```python
from build123d import *

# Parameters (mm, degrees)
SKETCH1_R               = 3
BOSS_EXTRUDE1_DEPTH     = 98.5
SKETCH2_R               = 4
BOSS_EXTRUDE2_DEPTH     = 4.7
SKETCH3_R               = 9
BOSS_EXTRUDE3_DEPTH     = 7.9
SKETCH4_R               = 5.9
BOSS_EXTRUDE4_DEPTH     = 8
SKETCH5_R               = 9
BOSS_EXTRUDE5_DEPTH     = 3
SKETCH6_R               = 1.4
CUT_EXTRUDE1_DEPTH      = 82
CUT_EXTRUDE1_DEPTH_BACK = 82
SKETCH7_R               = 3
SKETCH7_R_2             = 0.75
CUT_EXTRUDE2_DEPTH      = 9


with BuildPart() as part:
    # Sketch1 → Boss-Extrude1 (new body)
    with BuildSketch(Plane.XY):
        Circle(SKETCH1_R)
    extrude(amount=BOSS_EXTRUDE1_DEPTH)

    # Sketch2 → Boss-Extrude2 (add)
    with BuildSketch(Plane.XY.offset(98.5)):
        Circle(SKETCH2_R)
    extrude(amount=BOSS_EXTRUDE2_DEPTH)

    # Sketch3 → Boss-Extrude3 (add)
    with BuildSketch(Plane.XY.offset(103.2)):
        Circle(SKETCH3_R)
    extrude(amount=BOSS_EXTRUDE3_DEPTH)

    # Sketch4 → Boss-Extrude4 (add)
    with BuildSketch(Plane.XY.offset(111.1)):
        Circle(SKETCH4_R)
    extrude(amount=BOSS_EXTRUDE4_DEPTH)

    # Sketch5 → Boss-Extrude5 (add)
    with BuildSketch(Plane.XY.offset(119.1)):
        Circle(SKETCH5_R)
    extrude(amount=BOSS_EXTRUDE5_DEPTH)

    # Sketch6 → Cut-Extrude1 (cut, two sides)
    with BuildSketch(Plane(origin=(0, 0, 0), x_dir=(1, 0, 0), z_dir=(0, 1, 0))) as cut_extrude1_sk:
        with Locations((0, -40.4)):
            Circle(SKETCH6_R)
    extrude(amount=CUT_EXTRUDE1_DEPTH, mode=Mode.SUBTRACT)
    extrude(cut_extrude1_sk.sketch, amount=-CUT_EXTRUDE1_DEPTH_BACK, mode=Mode.SUBTRACT)

    # Sketch7 → Cut-Extrude2 (cut)
    with BuildSketch(Plane.XY.offset(122.1)):
        Circle(SKETCH7_R)
        with Locations((1.637751338, 7.588247864)):
            Circle(SKETCH7_R_2)
    extrude(amount=-CUT_EXTRUDE2_DEPTH, mode=Mode.SUBTRACT)


solid = part.part
```
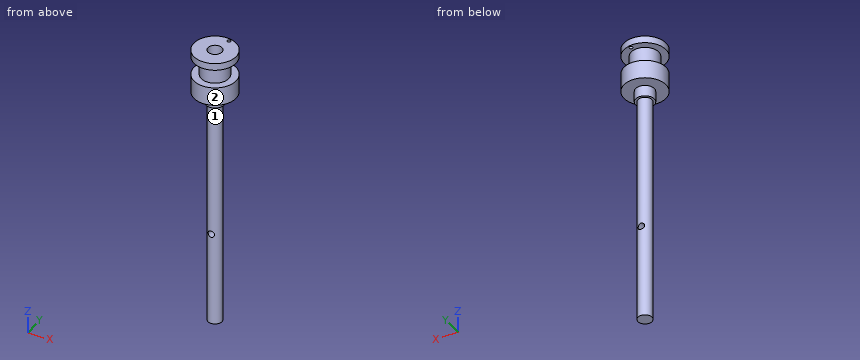
Model file for the job. Use its own axes, mm. Face numbers are marked on the shaded views. A direction names the side the tool comes from. Round coordinates to 2 decimals unless told otherwise and drop trailing zeros. Write each loop counter-clockwise with the first axis right and the second up, starting at its lowest first coordinate (ties: lowest second). Pieces come first, ordered by that corner, then holes. Notation, with made-up numbers: M -6,88 L 25,88 A17 cw 25,120 Z; hole C 51.25,84 d11. An arc over 180 degrees is marked long. Put each result on its own line as item: value.
Item 1: Cut at B-B (y = -1). List the corners of the cut face in (x, z), and give its area (3 significant figures).
Responses:
outline: M -8.94,103.2 L -3.87,103.2 L -3.87,98.5 L -2.83,98.5 L -2.83,0 L 2.83,0 L 2.83,98.5 L 3.87,98.5 L 3.87,103.2 L 8.94,103.2 L 8.94,111.1 L 5.81,111.1 L 5.81,119.1 L 8.94,119.1 L 8.94,122.1 L 2.83,122.1 L 2.83,113.1 L -2.83,113.1 L -2.83,122.1 L -8.94,122.1 L -8.94,119.1 L -5.81,119.1 L -5.81,111.1 L -8.94,111.1 Z; hole C 0,40.4 d2.8
area: 825 mm²
Item 2: Tool access for the marked faces 1 and 2: list every direction of +Z, -Z, +X, -X, +Y, -Y with a clear straight run to the whole face (end or side of a thin tool).
Responses:
face 1: -Z
face 2: +Z, -Z
Item 3: Probe L1, parallel to Z at x = 4.75, y = 7.25; L2, parallel to Y at x = 0, z = 52; L3, parallel to Z at x = -3.5, y = -4. List the from-to ranges inside material, lowest first. Write a range as from..to.
Responses:
L1: 103.2..111.1, 119.1..122.1
L2: -3..3
L3: 103.2..122.1
Item 4: Cut at C-C (z = 104.5). List the corners of the cut face in (x, y), and give its area (3 significant figures).
Responses:
outline: C 0,0 d18
area: 254 mm²
Item 5: Flat gauge pins, fed straight in: P1, Ø1.5, axis at x = 0.5, z = 22, coming from the -Y side; P2, Ø5, axis at x = -5, y = 6, coming from the -Z side; P3, Ø1.4, axis at x = 1.64, y = 7.59, coming from the +Z side. Where does each tip first touch, or does it go through?
Responses:
P1: y = -3
P2: z = 103.2
P3: z = 111.1
Item 6: Cut at D-D (z = 40.4). List the corners of the cut face in (x, y).
Responses:
outline: M -1.4,-2.65 L -1.4,2.65 A3 ccw Z; M 1.4,-2.65 A3 ccw 1.4,2.65 Z
Item 7: Cut at A-A (x = -7.5). List the corners of the cut face in (y, z), and give its area (3 significant figures).
Responses:
outline: M -4.97,103.2 L 4.97,103.2 L 4.97,111.1 L -4.97,111.1 Z; M -4.97,119.1 L 4.97,119.1 L 4.97,122.1 L -4.97,122.1 Z
area: 108 mm²
